```python
from build123d import *

# Parameters (mm, degrees)
F0_W     = 80
F0_H     = 40
F0_R     = 2.5
F0_R_2   = 12.5
F0_R_3   = 2.25
F1_DEPTH = 3
F2_R     = 5


with BuildPart() as f1:
    # F0 (on Front) → F1 (new body)
    with BuildSketch(Plane.XZ):
        Rectangle(F0_W, F0_H)
        with Locations((-35, -15.260881)):
            Circle(F0_R, mode=Mode.SUBTRACT)
        with Locations((35.486974, -15.883215)):
            Circle(F0_R, mode=Mode.SUBTRACT)
        with Locations((-20, 0)):
            Circle(F0_R_2, mode=Mode.SUBTRACT)
        with Locations((-35, 15)):
            Circle(F0_R, mode=Mode.SUBTRACT)
        with Locations((15, 0)):
            Circle(F0_R_3, mode=Mode.SUBTRACT)
        with Locations((35.486974, 15)):
            Circle(F0_R, mode=Mode.SUBTRACT)
    extrude(amount=F1_DEPTH)

    # F2
    f2_edges = [f1.edges().sort_by_distance(p)[0] for p in [
        (-40, -1.5, 20),
        (40, -1.5, 20),
        (40, -1.5, -20),
        (-40, -1.5, -20),
    ]]
    fillet(f2_edges, radius=F2_R)


solid = f1.part
```
Source: CAD feature listing. Evaluate the final solid. Frame: model axes, mm. Round coordinates to 2 decimals unless told otherwise and drop trailing zeros. Loops run counter-clockwise (first coordinate to the right, second up) from the corner with the lowest first, then second, coordinate; pieces in that order, holes last. Notation, with made-up numbers: M 73.5,36.25 L 107.5,36.25 A20 ccw 107.5,72.25 Z; hole C 82,-19.5 d4. An arc over 180 degrees is marked long. Use a Markdown table: item, result. Add a question column.
1. Section query C-C on y = -0.8. Return the cut outline in (x, z).
2. Line query: line 1 (Z direction, x = -35, y = -0.7); line 2 (Z direction, x = 15, y = -1.5); line 3 (X direction, y = -0.45, z = -16.5). Output: solid intervals per line, ascending.
3. Section query A-A on x = 15. Return the cut outline in (y, z).
4. Section query B-B on z = 6. Return the cut outline in (x, y).
Reported:
| question | item | result |
|---|---|---|
| 1 | outline | M -40,-15 A5 ccw -35,-20 L 35,-20 A5 ccw 40,-15 L 40,15 A5 ccw 35,20 L -35,20 A5 ccw -40,15 Z; hole C -35,-15.26 d5; hole C -35,15 d5; hole C -20,0 d25; hole C 15,0 d4.5; hole C 35.49,-15.88 d5; hole C 35.49,15 d5 |
| 2 | line 1 | z = -20 to -17.76, -12.76 to 12.5, 17.5 to 20 |
| 2 | line 2 | z = -20 to -2.25, 2.25 to 20 |
| 2 | line 3 | x = -39.77 to -37.17, -32.83 to 33.06, 37.91 to 39.77 |
| 3 | outline | M -3,-20 L 0,-20 L 0,-2.25 L -3,-2.25 Z; M -3,2.25 L 0,2.25 L 0,20 L -3,20 Z |
| 4 | outline | M -40,-3 L -30.97,-3 L -30.97,0 L -40,0 Z; M -9.03,-3 L 40,-3 L 40,0 L -9.03,0 Z |
